Can you work these out from the model? Positions are in its coordinate system, mm. Face numbers are marked on the shaded views. A direction names the side the tool comes from. Give positions to 0.01 mm unless a question says otherwise; leave off trailing zeros. Loops run counter-clockwise (first coordinate to the right, second up) from the corner with the lowest first, then second, coordinate; pieces in that order, holes last. Notation, with made-up numbers: (-15.5, 62) -> (32.5, 62) arc R28 cw to (32.5, 95) -> close; hole circle Ø8 at (56, -3). An arc over 180 degrees is marked (long way). One line per question, with ' | ' between items.
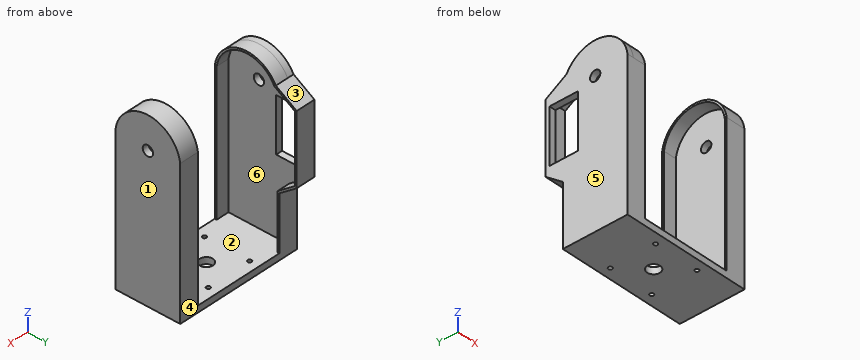
from build123d import *

# Parameters (mm, degrees)
SKETCH1_W           = 99
SKETCH1_H           = 50
BOSS_EXTRUDE1_DEPTH = 5
SKETCH2_W           = 5
SKETCH2_H           = 50
BOSS_EXTRUDE2_DEPTH = 130
SKETCH3_OUTSIDE_W   = 171.944
SKETCH3_OUTSIDE_H   = 86.944
SKETCH3_OUTSIDE_R   = 4
CUT_EXTRUDE1_DEPTH  = 170.266063
EXTRUDE_THIN2_DEPTH = 15
CUT_EXTRUDE3_REACH  = 171.266
SKETCH8_W           = 42.955183
SKETCH8_H           = 22
BOSS_EXTRUDE4_START = -5
BOSS_EXTRUDE4_DEPTH = 5
EXTRUDE_THIN3_START = -15
EXTRUDE_THIN3_DEPTH = 15
CUT_EXTRUDE5_REACH  = 150.819
SKETCH13_R          = 5
SKETCH5_R           = 1.5
CUT_EXTRUDE6_DEPTH  = 149.819085


with BuildPart() as part:
    # Sketch1 → Boss-Extrude1 (new body)
    with BuildSketch(Plane.XY):
        Rectangle(SKETCH1_W, SKETCH1_H)
    extrude(amount=BOSS_EXTRUDE1_DEPTH)

    # Sketch2 → Boss-Extrude2 (add)
    with BuildSketch(Plane.XY.offset(5)):
        with Locations((47, 0)):
            Rectangle(SKETCH2_W, SKETCH2_H)
        with Locations((-47, 0)):
            Rectangle(SKETCH2_W, SKETCH2_H)
    extrude(amount=BOSS_EXTRUDE2_DEPTH)

    # Sketch3 outside → Cut-Extrude1 (cut, through all)
    # profile 1 of 2: a face of its own
    with BuildSketch(Plane(origin=(49.5, 0, 0), x_dir=(0, 0, -1), z_dir=(1, 0, 0))):
        with Locations((-67.5, 0)):
            Rectangle(SKETCH3_OUTSIDE_W, SKETCH3_OUTSIDE_H)
        with BuildLine():
            Line((0, -25), (0, 25))
            Line((0, 25), (-106.5, 25))
            ThreePointArc((-106.5, 25), (-135, 0), (-106.5, -25))
            Line((-106.5, -25), (0, -25))
        make_face(mode=Mode.SUBTRACT)
    # profile 2 of 2: a face of its own
    with BuildSketch(Plane(origin=(49.5, 0, 0), x_dir=(0, 0, -1), z_dir=(1, 0, 0))):
        with Locations((-109.785088, 0)):
            Circle(SKETCH3_OUTSIDE_R)
    extrude(amount=-CUT_EXTRUDE1_DEPTH, mode=Mode.SUBTRACT)

    # Sketch7 → Extrude-Thin2 (add)
    with BuildSketch(Plane(origin=(49.5, 0, 0), x_dir=(0, 0, -1), z_dir=(1, 0, 0))):
        with BuildLine():
            Line((-113.070175, -25), (0, -25))
            Line((0, -25), (0, 25))
            Line((0, 25), (-113.070175, 25))
            ThreePointArc((-113.070175, 25), (-135, 0), (-113.070175, -25))
        make_face()
        with BuildLine():
            Line((-112.970533, -23.5), (-1.5, -23.5))
            Line((-1.5, -23.5), (-1.5, 23.5))
            Line((-1.5, 23.5), (-112.970533, 23.5))
            ThreePointArc((-112.970533, 23.5), (-133.5, 0), (-112.970533, -23.5))
        make_face(mode=Mode.SUBTRACT)
    extrude(amount=-EXTRUDE_THIN2_DEPTH)

    # Sketch8 → Cut-Extrude3 (cut, up to next)
    with BuildSketch(Plane.ZY.offset(49.5), mode=Mode.PRIVATE) as cut_extrude3_sk1:
        with Locations((84.477591, 24.364958)):
            Rectangle(SKETCH8_W, SKETCH8_H)
    cut_extrude3_tool1 = extrude(cut_extrude3_sk1.sketch, amount=-CUT_EXTRUDE3_REACH, mode=Mode.PRIVATE) & part.part
    add(cut_extrude3_tool1.solids().sort_by_distance((-49.5, 24.364958, 84.477592))[0], mode=Mode.SUBTRACT)

    # Sketch9 → Boss-Extrude4 (add)
    with BuildSketch(Plane.ZY.offset(49.5).offset(BOSS_EXTRUDE4_START)):
        with BuildLine():
            Line((121.7, 22.222211), (111.7, 38.364958))
            Line((111.7, 38.364958), (105.455183, 38.364958))
            Line((105.455183, 38.364958), (63.5, 38.364958))
            Line((63.5, 38.364958), (57.3, 38.364958))
            Line((57.3, 38.364958), (47.3, 25))
            Line((47.3, 25), (59.748378, 25))
            Line((59.748378, 25), (63, 25))
            Line((63, 25), (63, 13.364958))
            Line((63, 13.364958), (63.5, 13.364958))
            Line((63.5, 13.364958), (63.5, 35.320141))
            Line((63.5, 35.320141), (105.455183, 35.320141))
            Line((105.455183, 35.320141), (105.455183, 13.364958))
            Line((105.455183, 13.364958), (105.955183, 13.364958))
            Line((105.955183, 13.364958), (105.955183, 25))
            Line((105.955183, 25), (113.070175, 25))
            ThreePointArc((113.070175, 25), (117.510955, 24.002141), (121.7, 22.222211))
        make_face()
    extrude(amount=BOSS_EXTRUDE4_DEPTH)

    # Sketch12 → Extrude-Thin3 (add)
    with BuildSketch(Plane.ZY.offset(49.5).offset(EXTRUDE_THIN3_START)):
        with BuildLine():
            Line((121.7, 22.222211), (111.7, 38.364958))
            Line((111.7, 38.364958), (57.3, 38.364958))
            Line((57.3, 38.364958), (47.3, 25))
            Line((47.3, 25), (0, 25))
            Line((0, 25), (0, -25))
            Line((0, -25), (113.070175, -25))
            ThreePointArc((113.070175, -25), (134.589206, -4.532935), (121.7, 22.222211))
        make_face()
        with BuildLine():
            Line((120.640171, 21.084692), (110.864718, 36.864958))
            Line((110.864718, 36.864958), (58.051066, 36.864958))
            Line((58.051066, 36.864958), (48.051066, 23.5))
            Line((48.051066, 23.5), (1.5, 23.5))
            Line((1.5, 23.5), (1.5, -23.5))
            Line((1.5, -23.5), (112.970533, -23.5))
            ThreePointArc((112.970533, -23.5), (133.156712, -4.020481), (120.640171, 21.084692))
        make_face(mode=Mode.SUBTRACT)
    extrude(amount=EXTRUDE_THIN3_DEPTH)

    # Sketch13 → Cut-Extrude5 (cut, up to next)
    with BuildSketch(Plane(origin=(0, 0, 0), x_dir=(-1, 0, 0), z_dir=(0, 0, -1)), mode=Mode.PRIVATE) as cut_extrude5_sk1:
        Circle(SKETCH13_R)
    cut_extrude5_tool1 = extrude(cut_extrude5_sk1.sketch, amount=-CUT_EXTRUDE5_REACH, mode=Mode.PRIVATE) & part.part
    add(cut_extrude5_tool1.solids().sort_by_distance((0, 0, 0))[0], mode=Mode.SUBTRACT)

    # Sketch5 → Cut-Extrude6 (cut, through all)
    with BuildSketch(Plane(origin=(0, 0, 0), x_dir=(-1, 0, 0), z_dir=(0, 0, -1))):
        with Locations((17.5, 17.5)):
            Circle(SKETCH5_R)
        with Locations((17.5, -17.5)):
            Circle(SKETCH5_R)
        with Locations((-17.5, -17.5)):
            Circle(SKETCH5_R)
        with Locations((-17.5, 17.5)):
            Circle(SKETCH5_R)
    extrude(amount=-CUT_EXTRUDE6_DEPTH, mode=Mode.SUBTRACT)


solid = part.part
Q1. If we mould it in two halves opening along Y, with no side actions, what happens to the marked faces 1, 2 and 3? For each: pulls with the +Y half, pulls with the -Y half, needs draft (parallel to the pull), parting line crosses it, or undercut.
Entries:
face 1: needs draft | face 2: undercut | face 3: pulls with the +Y half
Q2. On a 3-axis mill with a long thin cutter (end or side, diameter ignored), from which of +Z, -Z, +X, -X, +Y, -Y can I reach the whole of each face in a straight line? I mean the marked faces 4, 5 and 6. Say none if no direction works.
Entries:
face 4: -Z, +X, +Y | face 5: +Z, -Z, -X, +Y, -Y | face 6: none
Q3. For pin 1 Ø5 at (x, z) = (42, 47.5) entering from +Y; pin 2 Ø11 at (x, z) = (-42, 51.5) entering from +Y; pin 3 Ø2.5 at (x, y) = (-48, 24) entering from +Z, each with a flat end and sliding along its axis, tell me the tip position at first contact or that it passes through.
Entries:
pin 1: y = 25 | pin 2: y = 37.96 | pin 3: z = 121.37
Q4. If we section it at B-B (z = 104): Write out the boundary of the cut face in (x, y).
Entries:
outline: (-49.5, -25) -> (-34.5, -25) -> (-34.5, -23.5) -> (-44.5, -23.5) -> (-44.5, 13.36) -> (-49.5, 13.36) -> close; (-49.5, 35.32) -> (-44.5, 35.32) -> (-44.5, 36.86) -> (-34.5, 36.86) -> (-34.5, 38.36) -> (-49.5, 38.36) -> close; (34.5, -25) -> (49.5, -25) -> (49.5, 25) -> (34.5, 25) -> (34.5, 23.5) -> (44.5, 23.5) -> (44.5, -23.5) -> (34.5, -23.5) -> close
Q5. If we section it at A-A (x = 0): Write out the boundary of the cut face in (y, z).
Entries:
outline: (-25, 0) -> (-5, 0) -> (-5, 5) -> (-25, 5) -> close; (5, 0) -> (25, 0) -> (25, 5) -> (5, 5) -> close
Q6. If we section it at D-D (z = 23): Write out the boundary of the cut face in (x, y), plus the area to 3 significant figures.
Entries:
outline: (-49.5, -25) -> (-34.5, -25) -> (-34.5, -23.5) -> (-44.5, -23.5) -> (-44.5, 23.5) -> (-34.5, 23.5) -> (-34.5, 25) -> (-49.5, 25) -> close; (34.5, -25) -> (49.5, -25) -> (49.5, 25) -> (34.5, 25) -> (34.5, 23.5) -> (44.5, 23.5) -> (44.5, -23.5) -> (34.5, -23.5) -> close | area: 560 mm²
Q7. If we section it at C-C (y = 0): Write out the boundary of the cut face in (x, z), plus the area to 4 significant figures.
Entries:
outline: (-49.5, 0) -> (-5, 0) -> (-5, 5) -> (-44.5, 5) -> (-44.5, 105.79) -> (-49.5, 105.79) -> close; (-49.5, 113.79) -> (-44.5, 113.79) -> (-44.5, 133.5) -> (-34.5, 133.5) -> (-34.5, 135) -> (-49.5, 135) -> close; (5, 0) -> (49.5, 0) -> (49.5, 105.79) -> (44.5, 105.79) -> (44.5, 5) -> (5, 5) -> close; (34.5, 133.5) -> (44.5, 133.5) -> (44.5, 113.79) -> (49.5, 113.79) -> (49.5, 135) -> (34.5, 135) -> close | area: 1,695 mm²
Q8. If I drill on probe 1 along Y at (x, z) = (-17.5, 3.5); probe 2 along X at (y, z) = (-9.5, 122.5); probe 3 along X at (y, z) = (-17, 3), over which ranges is the centre line in solid material (lowest first)? Write a range as from..to.
Entries:
probe 1: -25..-19, -16..16, 19..25 | probe 2: -49.5..-44.5, 44.5..49.5 | probe 3: -49.5..-18.91, -16.09..16.09, 18.91..49.5
